The model under review builds one solid part; all positions refer to its coordinate system, in mm. A direction names the side the tool comes from. Give positions to 0.01 mm unless a question says otherwise; leave off trailing zeros. Order: outer loops, then holes, each group sorted by start corner. A loop starts at its lowest first (then second) coordinate and runs counter-clockwise, first axis right, second up.
```python
from build123d import *

# Parameters (mm, degrees)
SKETCH_1_R      = 1.6
SKETCH_1_R_2    = 1.6000000000000019
EXTRUDE_1_DEPTH = 5
SKETCH_2_R      = 1.6000000000000016
SKETCH_2_R_2    = 1.6000000000000125
SKETCH_2_R_3    = 1.6000000000000019
EXTRUDE_2_DEPTH = 3
CHAMFER_1_SIZE  = 0.5


with BuildPart() as part:
    # 草图1 → 凸台-拉伸1 (new body)
    with BuildSketch(Plane.XY):
        with BuildLine():
            Line((0, 2.000000000000014), (0, 19.705362587260357))
            ThreePointArc((0, 19.705362587260357), (-0.4134107583503983, 22.243799838501072), (-1.610915919621628, 24.519882772476706))
            Line((-1.610915919621628, 24.519882772476706), (-1.9727102009459283, 25))
            Line((-1.9727102009459283, 25), (13.999999999999998, 37.036300463040874))
            Line((13.999999999999998, 37.036300463040874), (18.389084080378368, 31.211789162518105))
            ThreePointArc((18.389084080378368, 31.211789162518105), (19.586589241649598, 28.93570622854247), (19.999999999999993, 26.397268977301756))
            Line((19.999999999999993, 26.397268977301756), (20, 2.0000000000000147))
            ThreePointArc((20, 2.0000000000000147), (19.414213562373096, 0.5857864376269051), (17.999999999999986, 0))
            Line((17.999999999999986, 0), (2.000000000000014, 0))
            ThreePointArc((2.000000000000014, 0), (0.5857864376269044, 0.5857864376269049), (0, 2.000000000000014))
        make_face()
        with Locations((5.299999999999996, 16)):
            Circle(SKETCH_1_R, mode=Mode.SUBTRACT)
        with Locations((17.3, 3.999999999999999)):
            Circle(SKETCH_1_R_2, mode=Mode.SUBTRACT)
    extrude(amount=EXTRUDE_1_DEPTH)

    # 草图2 → 凸台-拉伸2 (add)
    with BuildSketch(Plane(origin=(-12.730249987910918, 16.89361232439068, 0), x_dir=(0.7986355100472964, 0.6018150231520436, 0), z_dir=(-0.6018150231520436, 0.7986355100472964, 0))):
        with BuildLine():
            Line((30.96989916129314, -11.000000000000002), (15.969899161293144, -11.000000000000002))
            ThreePointArc((15.969899161293144, -11.000000000000002), (14.202132208326773, -10.267766952966369), (13.469899161293144, -8.499999999999998))
            Line((13.469899161293144, -8.499999999999998), (13.469899161293144, 3.500000000000003))
            ThreePointArc((13.469899161293144, 3.500000000000003), (14.202132208326775, 5.267766952966372), (15.969899161293144, 6.000000000000004))
            Line((15.969899161293144, 6.000000000000004), (30.96989916129314, 6.000000000000004))
            ThreePointArc((30.96989916129314, 6.000000000000004), (32.737666114259504, 5.26776695296637), (33.469899161293135, 3.5000000000000036))
            Line((33.469899161293135, 3.5000000000000036), (33.469899161293135, -8.499999999999998))
            ThreePointArc((33.469899161293135, -8.499999999999998), (32.73766611425951, -10.267766952966369), (30.96989916129314, -11.000000000000002))
        make_face()
        with Locations((17.21989916129313, 3.0000000000000004)):
            Circle(SKETCH_2_R, mode=Mode.SUBTRACT)
        with Locations((29.71989916129313, 3.0000000000000018)):
            Circle(SKETCH_2_R_2, mode=Mode.SUBTRACT)
        with Locations((29.71989916129313, -7.999999999999998)):
            Circle(SKETCH_2_R_2, mode=Mode.SUBTRACT)
        with Locations((17.21989916129313, -8)):
            Circle(SKETCH_2_R_3, mode=Mode.SUBTRACT)
    extrude(amount=EXTRUDE_2_DEPTH)

    # 倒角1
    chamfer_1_edges = [part.edges().sort_by_distance(p)[0] for p in [
        (-0.4134107583503974, 22.243799838501072, 5),
        (19.999999999999996, 14.198634488650885, 0),
        (19.414213562373096, 0.5857864376269046, 0),
        (10, 0, 0),
        (0.5857864376269049, 0.5857864376269046, 0),
        (0, 10.852681293630186, 0),
        (-0.4134107583503974, 22.243799838501072, 0),
        (-1.7918130602837783, 24.759941386238353, 0),
        (0, 10.852681293630186, 5),
        (0.5857864376269049, 0.5857864376269046, 5),
        (10, 0, 5),
        (19.414213562373096, 0.5857864376269046, 5),
        (19.999999999999996, 14.198634488650885, 5),
        (19.586589241649598, 28.93570622854247, 5),
        (16.194542040189184, 34.12404481277949, 5),
        (-3.19336795741086, 27.83657537829513, 10.267766952966369),
        (4.208199830070912, 33.41405676166233, 11.000000000000002),
        (11.609767617552686, 38.99153814502953, 10.26776695296637),
        (12.194554930543871, 39.43220699318276, 2.4999999999999973),
        (11.609767617552682, 38.99153814502952, -5.26776695296637),
        (4.208199830070912, 33.41405676166233, -6.000000000000004),
        (-3.1933679574108584, 27.83657537829513, -5.267766952966372),
        (-3.778155270402049, 27.395906530141897, 2.4999999999999973),
        (-1.3879228879547298, 25.440668848153244, 10.267766952966369),
        (6.013644899527042, 31.018150231520444, 11.000000000000002),
        (13.415212687008816, 36.59563161488764, 10.26776695296637),
        (14.000000000000002, 37.036300463040874, 6.75),
        (14.000000000000002, 37.036300463040874, -1.7500000000000018),
        (13.415212687008813, 36.59563161488764, -5.26776695296637),
        (6.013644899527042, 31.018150231520444, -6.000000000000004),
        (-1.387922887954728, 25.440668848153244, -5.267766952966372),
        (-1.9727102009459188, 25.000000000000007, -1.7500000000000018),
        (-1.9727102009459188, 25.000000000000007, 6.749999999999999),
        (-1.7918130602837783, 24.759941386238353, 5),
        (16.194542040189184, 34.12404481277949, 0),
        (19.586589241649598, 28.93570622854247, 0),
    ]]
    chamfer(chamfer_1_edges, length=CHAMFER_1_SIZE)


solid = part.part
```
1. Take a section at A-A (y = 4). Write out the cut boundary in (x, z), and give its area (3 significant figures).
2. Take a section at C-C (z = -1). Write out the cut boundary in (x, y).
3. Take a section at D-D (x = 5.3). Write out the cut boundary in (y, z), and give its area (3 significant figures).
4. Take a section at B-B (z = 2.5). Write out the cut boundary in (x, y).
5. For faces 1 (the flat face through (11, 15, 0)), 2 (the flat face through (-1.662, 25.008, 0.246)), 3 (the flat face through (11, 15, 5)), list the 3-axis set-ups (+Z, -Z, +X, -X, +Y, -Y) from which the entire face can be reached by the end or side of a thin tool; tool diameter is ignored.
6. To check wall thickness, follow line 1 (Z direction, x = 8.5, y = 28); line 2 (Y direction, x = 17.3, z = 2.1); line 3 (X direction, y = 8.5, z = 2.75). State the ranges of each line that lie inside material, in increasing order.
7. Insertion check: pin 1 (10.5 mm diameter, centred on x = 10, y = 15, fed in from +Z); pin 2 (2 mm diameter, centred on y = 10, z = 1.5, fed in from -X); pin 3 (3 mm diameter, centred on x = 8, y = 5.5, fed in from -Z); pin 4 (2.5 mm diameter, centred on x = 5.3, y = 16, fed in from -Z). Each pin has a flat end and moves straight along its axis. Give the tip position at first contact, or say it passes through.
8. Draft analysis for pull direction Z (two halves, no side actions). For faces 4 (the flat face through (20, 14, 2)), 5 (the conical face through (0.85, 0.83, 4.86)), 6 (the cylindrical face through (-0.145, 28.229, 9.562)), 7 (the cylindrical face through (11.334, 36.879, -3.481)), state which applies: pulls with the +Z half, pulls with the -Z half, needs draft (parallel to the pull), parting line crosses it, or undercut.
Answer:
1. outline: (0, 0.5) - (0.5, 0) - (15.7, 0) - (15.7, 5) - (0.5, 5) - (0, 4.5) - close; (18.9, 0) - (19.5, 0) - (20, 0.5) - (20, 4.5) - (19.5, 5) - (18.9, 5) - close
1. area: 83.5 mm2
2. outline: (-3.48, 27) - (-2.27, 25.4) - (-1.57, 25.3) - (13.6, 36.74) - (13.7, 37.44) - (12.5, 39.03) - (11.8, 39.13) - (-3.38, 27.7) - close
3. outline: (0, 0.5) - (0.5, 0) - (14.4, 0) - (14.4, 5) - (0.5, 5) - (0, 4.5) - close; (17.6, 0) - (30.48, 0) - (30.48, -5.5) - (31.11, -6) - (33.61, -6) - (34.24, -5.5) - (34.24, 10.5) - (33.61, 11) - (31.11, 11) - (30.48, 10.5) - (30.48, 5) - (17.6, 5) - close
3. area: 199 mm2
4. outline: (-3.48, 27) - (-1.61, 24.52) arc R8 cw to (0, 19.71) - (0, 2) arc R2 ccw to (2, 0) - (18, 0) arc R2 ccw to (20, 2) - (20, 26.4) arc R8 ccw to (18.39, 31.21) - (12.5, 39.03) - (11.8, 39.13) - (-3.38, 27.7) - close; hole circle Ø3.2 at (5.3, 16); hole circle Ø3.2 at (17.3, 4)
5. face 1: -Z, +X, -Y
5. face 2: -Z, -X, -Y
5. face 3: +Z, +X, -Y
6. line 1: z = 0 to 5
6. line 2: y = 0 to 2.4, 5.6 to 32.66
6. line 3: x = 0 to 20
7. pin 1: stops at z = 5
7. pin 2: stops at x = 0
7. pin 3: stops at z = 0
7. pin 4: passes through
8. face 4: needs draft
8. face 5: pulls with the +Z half
8. face 6: undercut
8. face 7: undercut
